Verification items for the finished model (mm, model axes). A direction names the side the tool comes from. Give positions to 0.01 mm unless a question says otherwise; leave off trailing zeros. Order: outer loops, then holes, each group sorted by start corner. A loop starts at its lowest first (then second) coordinate and runs counter-clockwise, first axis right, second up. Notation, with made-up numbers: M 34.25,39.5 L 54.25,39.5 A5 cw 54.25,44.5 Z; hole C 67.5,67 d4. An arc over 180 degrees is marked long. Answer as a JSON object with one key per item and string values.
```python
from build123d import *

# Parameters (mm, degrees)
SKETCH1_R           = 36.25
BOSS_EXTRUDE1_DEPTH = 3
SKETCH2_R           = 1.5
CUT_EXTRUDE1_DEPTH  = 52.352945388
SKETCH3_R           = 4
CUT_EXTRUDE2_DEPTH  = 8
CIRPATTERN1_COUNT   = 6
SKETCH4_R           = 1.5
CUT_EXTRUDE3_DEPTH  = 52.352945388
CIRPATTERN2_COUNT   = 6


with BuildPart() as part:
    # Sketch1 → Boss-Extrude1 (new body)
    with BuildSketch(Plane(origin=(0, 0, 0), x_dir=(1, 0, 0), z_dir=(0, 1, 0))):
        with Locations(Location((0, 0, 0), (0, 0, 270))):
            Circle(SKETCH1_R)
    extrude(amount=BOSS_EXTRUDE1_DEPTH)

    # Sketch2 → Cut-Extrude1 (cut, symmetric)
    with BuildSketch(Plane(origin=(0, 3, 0), x_dir=(1, 0, 0), z_dir=(0, 1, 0))):
        with Locations(Location((0, 33.25, 0), (0, 0, 270))):
            Circle(SKETCH2_R)
    cut_extrude1 = extrude(amount=CUT_EXTRUDE1_DEPTH, both=True, mode=Mode.SUBTRACT)

    # Sketch3 → Cut-Extrude2 (cut)
    with BuildSketch(Plane(origin=(0, 3, 0), x_dir=(1, 0, 0), z_dir=(0, 1, 0))):
        with Locations(Location((0, 0, 0), (0, 0, 270))):
            Circle(SKETCH3_R)
        with BuildLine():
            Line((-5, 24.494897428), (-5, 13.076696831))
            ThreePointArc((-5, 13.076696831), (-9.899494937, 9.899494937), (-13.076696831, 5))
            Line((-13.076696831, 5), (-24.494897428, 5))
            ThreePointArc((-24.494897428, 5), (-17.67766953, 17.67766953), (-5, 24.494897428))
        make_face()
        with BuildLine():
            Line((5, 24.494897428), (5, 13.076696831))
            ThreePointArc((5, 13.076696831), (9.899494937, 9.899494937), (13.076696831, 5))
            Line((13.076696831, 5), (24.494897428, 5))
            ThreePointArc((24.494897428, 5), (17.67766953, 17.67766953), (5, 24.494897428))
        make_face()
        with BuildLine():
            Line((24.494897428, -5), (13.076696831, -5))
            ThreePointArc((13.076696831, -5), (9.899494937, -9.899494937), (5, -13.076696831))
            Line((5, -13.076696831), (5, -24.494897428))
            ThreePointArc((5, -24.494897428), (17.67766953, -17.67766953), (24.494897428, -5))
        make_face()
        with BuildLine():
            Line((-5, -24.494897428), (-5, -13.076696831))
            ThreePointArc((-5, -13.076696831), (-9.899494937, -9.899494937), (-13.076696831, -5))
            Line((-13.076696831, -5), (-24.494897428, -5))
            ThreePointArc((-24.494897428, -5), (-17.67766953, -17.67766953), (-5, -24.494897428))
        make_face()
    extrude(amount=-CUT_EXTRUDE2_DEPTH, mode=Mode.SUBTRACT)

    # CirPattern1: Cut-Extrude1 ×6 about axis
    cirpattern1_axis = Axis((0, 0, 0), (0, 1, 0))
    for i in range(1, CIRPATTERN1_COUNT):
        add(cut_extrude1.rotate(cirpattern1_axis, i * 360 / CIRPATTERN1_COUNT), mode=Mode.SUBTRACT)

    # Sketch4 → Cut-Extrude3 (cut, through all)
    with BuildSketch(Plane(origin=(0, 3, 0), x_dir=(1, 0, 0), z_dir=(0, 1, 0))):
        with Locations(Location((0, 10.5, 0), (0, 0, 270))):
            Circle(SKETCH4_R)
    cut_extrude3 = extrude(amount=-CUT_EXTRUDE3_DEPTH, mode=Mode.SUBTRACT)

    # CirPattern2: Cut-Extrude3 ×6 about axis
    cirpattern2_axis = Axis((0, 0, 0), (0, 1, 0))
    for i in range(1, CIRPATTERN2_COUNT):
        add(cut_extrude3.rotate(cirpattern2_axis, i * 360 / CIRPATTERN2_COUNT), mode=Mode.SUBTRACT)


solid = part.part
```
Q1. Section check D-D on y = 1.45. Count the separate pieces of the cut face and the enclosed holes in it, then the cut area to 3 significant figures.
Resolved:
{"separate pieces": "1", "enclosed holes": "17", "area": "3,090 mm²"}
Q2. Section check A-A on x = 0. Record the cut outline in (y, z).
Resolved:
{"outline": "M 0,-36.25 L 3,-36.25 L 3,-34.75 L 0,-34.75 Z; M 0,-31.75 L 3,-31.75 L 3,-12 L 0,-12 Z; M 0,-9 L 3,-9 L 3,-4 L 0,-4 Z; M 0,4 L 3,4 L 3,9 L 0,9 Z; M 0,12 L 3,12 L 3,31.75 L 0,31.75 Z; M 0,34.75 L 3,34.75 L 3,36.25 L 0,36.25 Z"}
Q3. Release check for a two-part mould opening along Z. For faces 3 (the face through (1, 3, 8)), 4 (the face through (5, 2, -19)), 5 (the face through (9.8, 1.5, -10)) record: +Z half, -Z half, draft (parallel to the pull), parting line (faces both ways), or undercut.
Resolved:
{"face 3": "draft", "face 4": "undercut", "face 5": "undercut"}
Q4. Section check B-B on z = -11. Record the cut outline in (x, y).
Resolved:
{"outline": "M -34.54,0 L -22.45,0 L -22.45,3 L -34.54,3 Z; M -8.66,0 L -1.41,0 L -1.41,3 L -8.66,3 Z; M 1.41,0 L 8.66,0 L 8.66,3 L 1.41,3 Z; M 22.45,0 L 34.54,0 L 34.54,3 L 22.45,3 Z"}
Q5. Tool access check on faces 1 (the face through (19, 2, 5)), 2 (the face through (1, 0, 8)). Record the directions out of +Z, -Z, +X, -X, +Y, -Y that give a thin tool (end or side, any length) a straight path to the whole face; none if there is none.
Resolved:
{"face 1": "+Y, -Y", "face 2": "+Z, -Z, +X, -X, -Y"}
Q6. Material ranges on L1, parallel to Z at x = -28.5, y = 2.7; L2, parallel to X at y = 2, z = -8; L3, parallel to X at y = 2.45, z = -14, recorded low to high.
Resolved:
{"L1": "z = -22.4 to -18.1, -15.15 to 15.15, 18.1 to 22.4", "L2": "x = -35.36 to -23.69, -11.49 to 11.49, 23.69 to 35.36", "L3": "x = -33.44 to -20.71, -5 to 5, 20.71 to 33.44"}
Q7. Gauge pin test, flat ends, axial feed: pin 1 Ø12 at (x, z) = (1, 16) entering from -Y; pin 2 Ø0.9 at (x, y) = (19.5, 2) entering from -Z; pin 3 Ø1.5 at (y, z) = (2, -21) entering from -X; pin 4 Ø0.9 at (x, y) = (-21, 2) entering from -Z. Record the tip position at first contact, or that the pin passes through.
Resolved:
{"pin 1": "stops at y = 0", "pin 2": "stops at z = -30.84", "pin 3": "stops at x = -30.07", "pin 4": "stops at z = -29.86"}
Q8. Section check C-C on x = -9. Record the cut outline in (y, z), then the cut area to 3 significant figures.
Resolved:
{"outline": "M 0,-35.11 L 3,-35.11 L 3,-23.32 L 0,-23.32 Z; M 0,-10.72 L 3,-10.72 L 3,-6.75 L 0,-6.75 Z; M 0,-3.75 L 3,-3.75 L 3,3.75 L 0,3.75 Z; M 0,6.75 L 3,6.75 L 3,10.72 L 0,10.72 Z; M 0,23.32 L 3,23.32 L 3,35.11 L 0,35.11 Z", "area": "117 mm²"}
